Geometry: final body of the model. Coordinates: model frame, mm. A direction names the side the tool comes from. Coordinates: 2 decimals unless noted, no trailing zeros. Order: outer loops, then holes, each group sorted by start corner. A loop starts at its lowest first (then second) coordinate and runs counter-clockwise, first axis right, second up. Notation, with made-up numbers: (-18.5, 11.25) -> (-8.5, 11.25) arc R7 cw to (-8.5, 15.25) -> close; hole circle Ø4 at (-34.5, 58.5). An arc over 180 degrees is marked (long way). Answer in a Markdown table with one row per item. Add a question column.
1) Contact query for a flat-ended pin moving along its axis: P1, Ø3, axis at y = -5, z = 2, coming from the -X side. Output: stop coordinate, or through.
2) Set-up query: faces 1 (the face through (40.242, -15.075, 0.044)), 2 (the face through (58.35, 13.167, -0.044)). Return all of +Z, -Z, +X, -X, +Y, -Y with unobstructed straight access to the full face (end or side cutting, diameter ignored); none if empty.
3) Pull-direction query (Y, two-part tool) for faces 3 (the face through (43, -2, 3.175)), 4 (the face through (56.36, -39.05, 0.04)), 5 (the face through (57.84, -23.31, -0.04)), 6 (the face through (8.6, 11.9, 0)); classes: +Y half, -Y half, draft (parallel to the pull), parting line (faces both ways), or undercut.
4) Section query B-B on x = 21.5. Return the cut outline in (y, z) (3 decimals), then the cut area to 3 significant figures.
5) Section query A-A on z = -2.25. Count the separate pieces of the cut face and the enclosed holes in it, then the cut area to 3 significant figures.
6) Ray query, line 1 (Y direction, x = 52.5, z = -1.5); line 2 (Y direction, x = 57, z = 2); line 3 (X direction, y = -20.5, z = 1). Return the intervals inside material, ascending. Write a range as from..to.
7) Section query C-C on y = 9. Return the cut outline in (x, z) (3 decimals), then the cut area to 3 significant figures.
```python
from build123d import *

# Parameters (mm, degrees)
SKETCH1_R           = 2.4892
BOSS_EXTRUDE1_DEPTH = 3.175
FILLET1_R           = 1.5875


with BuildPart() as part:
    # Sketch1 → Boss-Extrude1 (new, symmetric)
    with BuildSketch(Plane.XY):
        with BuildLine():
            ThreePointArc((18.812153865, -0.385081668), (15.640023815, 2.489031981), (13.351109218, 6.106186705))
            ThreePointArc((13.351109218, 6.106186705), (7.933835302, 12.352809027), (0, 14.6812))
            Line((0, 14.6812), (0, 27.3812))
            Line((0, 27.3812), (69.85, 27.3812))
            Line((69.85, 27.3812), (69.85, -48.8188))
            Line((69.85, -48.8188), (49.664583845, -48.8188))
            Line((49.664583845, -48.8188), (62.388915679, -30.256239225))
            Line((62.388915679, -30.256239225), (18.812153865, -0.385081668))
        make_face()
        with Locations((60.325, -23.4188)):
            Circle(SKETCH1_R, mode=Mode.SUBTRACT)
        with Locations((60.325, 14.6812)):
            Circle(SKETCH1_R, mode=Mode.SUBTRACT)
    extrude(amount=BOSS_EXTRUDE1_DEPTH, both=True)

    # Fillet1
    fillet1_edges = [part.edges().sort_by_distance(p)[0] for p in [
        (0, 14.6812, 0),
        (49.664583845, -48.8188, 0),
        (62.388915679, -30.256239225, 0),
    ]]
    fillet(fillet1_edges, radius=FILLET1_R)


solid = part.part
```
Result:
| question | item | result |
|---|---|---|
| 1 | P1 | x = 23.36 |
| 2 | face 1 | +Z, -Z, -X |
| 2 | face 2 | +Z, -Z |
| 3 | face 3 | draft |
| 3 | face 4 | undercut |
| 3 | face 5 | undercut |
| 3 | face 6 | -Y half |
| 4 | outline | (-2.228, -3.175) -> (27.381, -3.175) -> (27.381, 3.175) -> (-2.228, 3.175) -> close |
| 4 | area | 188 mm2 |
| 5 | separate pieces | 1 |
| 5 | enclosed holes | 2 |
| 5 | area | 2,850 mm2 |
| 6 | line 1 | -48.81..-44.68, -23.48..27.38 |
| 6 | line 2 | -48.82..-38.12, -26.56..27.38 |
| 6 | line 3 | 48.16..69.85 |
| 7 | outline | (11.599, -3.175) -> (69.85, -3.175) -> (69.85, 3.175) -> (11.599, 3.175) -> close |
| 7 | area | 370 mm2 |
